```python
from build123d import *

# Parameters (mm, degrees)
SKETCH1_W           = 120
SKETCH1_H           = 85
BOSS_EXTRUDE1_DEPTH = 45
SHELL1_T            = -3
SKETCH5_R           = 5
CUT_EXTRUDE2_DEPTH  = 45
FILLET1_R           = 2


with BuildPart() as part:
    # Sketch1 → Boss-Extrude1 (new body)
    with BuildSketch(Plane(origin=(0, 0, 0), x_dir=(1, 0, 0), z_dir=(0, 1, 0))):
        Rectangle(SKETCH1_W, SKETCH1_H)
    extrude(amount=BOSS_EXTRUDE1_DEPTH)

    # Shell1
    shell1_openings = [part.faces().sort_by_distance(p)[0] for p in [
        (0, 45, 0),
    ]]
    offset(amount=SHELL1_T, openings=shell1_openings, kind=Kind.INTERSECTION)

    # Sketch5 → Cut-Extrude2 (cut)
    with BuildSketch(Plane(origin=(0, 0, 39.5), x_dir=(-1, 0, 0), z_dir=(0, 0, -1))):
        with Locations((34.130287034, 18)):
            Circle(SKETCH5_R)
    extrude(amount=-CUT_EXTRUDE2_DEPTH, mode=Mode.SUBTRACT)

    # Fillet1
    fillet1_edges = [part.edges().sort_by_distance(p)[0] for p in [
        (0, 0, -42.5),
        (60, 0, 0),
        (0, 0, 42.5),
        (-60, 0, 0),
    ]]
    fillet(fillet1_edges, radius=FILLET1_R)


solid = part.part
```
Build history of the part. All positions in model axes, mm. A direction names the side the tool comes from. Round coordinates to 2 decimals unless told otherwise and drop trailing zeros. Loops run counter-clockwise (first coordinate to the right, second up) from the corner with the lowest first, then second, coordinate; pieces in that order, holes last.
Item 1: Saw through at C-C (y = 18). List the corners of the cut face in (x, z), then the cut area to 3 significant figures.
Item 2: Two-plate mould, pull along Z, no slides. Class faces 1 (the face through (-1, 3, -1)), 2 (the face through (-5, 45, 41)), 3 (the face through (-1, 23, 42.5)), 4 (the face through (-1, 24, 39.5)): released by +Z, released by -Z, zero draft, split by the parting line, or undercut.
Item 3: Saw through at A-A (x = 1). List the corners of the cut face in (y, z).
Item 4: Which spindle directions (+Z, -Z, +X, -X, +Y, -Y) get a long thin tool onto all of the face, cutting with end or side? Do faces 5 (the face through (-33.05, 13.12, 40.98)), 6 (the face through (60, 23, 1)), 7 (the face through (-57, 24, 1)). Say none if no direction does.
Item 5: Pin check, flat tip, straight feed: P1, Ø3, axis at x = 18, z = 20.5, coming from the +Y side. Stop position of the tip, or through.
Item 6: Drill centre lines: line 1 along X through (y, z) = (43.5, -9); line 2 along Z through (x, y) = (26, 17.5); line 3 along Y through (x, z) = (-53.5, 2). Where is each one in solid material? Low to high.
Item 7: Saw through at B-B (z = 30.5). List the corners of the cut face in (x, y).
Worked answers:
1. outline: (-60, -42.5) - (60, -42.5) - (60, 42.5) - (-29.13, 42.5) - (-29.13, 39.5) - (57, 39.5) - (57, -39.5) - (-57, -39.5) - (-57, 39.5) - (-39.13, 39.5) - (-39.13, 42.5) - (-60, 42.5) - close
1. area: 1,160 mm2
2. face 1: undercut
2. face 2: zero draft
2. face 3: released by +Z
2. face 4: undercut
3. outline: (0, -40.5) arc R2 ccw to (2, -42.5) - (45, -42.5) - (45, -39.5) - (3, -39.5) - (3, 39.5) - (45, 39.5) - (45, 42.5) - (2, 42.5) arc R2 ccw to (0, 40.5) - close
4. face 5: +Z
4. face 6: +Z, -Z, +X, +Y, -Y
4. face 7: +Y
5. P1: stops at y = 3
6. line 1: x = -60 to -57, 57 to 60
6. line 2: z = -42.5 to -39.5, 39.5 to 42.5
6. line 3: y = 0 to 3
7. outline: (-60, 2) arc R2 ccw to (-58, 0) - (58, 0) arc R2 ccw to (60, 2) - (60, 45) - (57, 45) - (57, 3) - (-57, 3) - (-57, 45) - (-60, 45) - close
